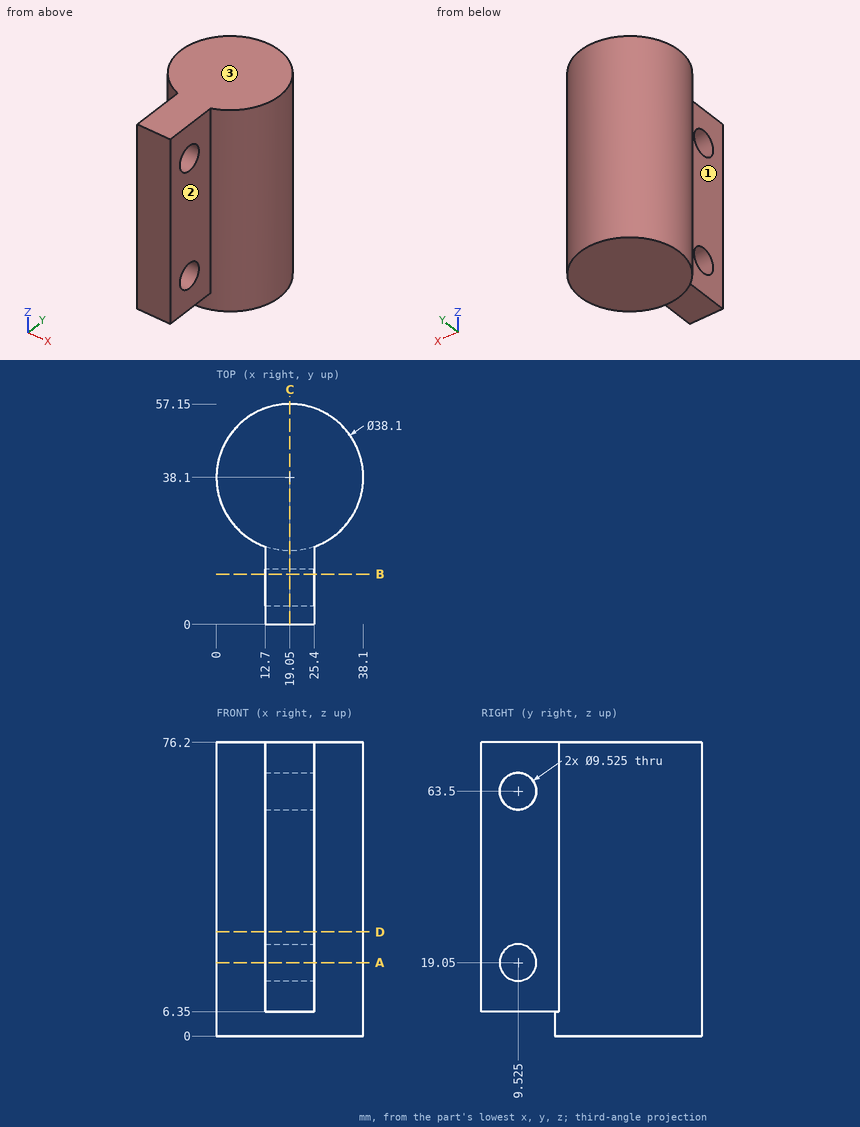
Part print with two shaded views. Sizes in mm from the minimum x, y, z corner. A direction names the side the tool comes from. Coordinates: 2 decimals unless noted, no trailing zeros. Loops run counter-clockwise (first coordinate to the right, second up) from the corner with the lowest first, then second, coordinate; pieces in that order, holes last. Notation, with made-up numbers: (39.25, 65.25) - (64.25, 65.25) arc R20 ccw to (64.25, 78.25) - close; hole circle Ø1 at (79.5, 49). An arc over 180 degrees is marked (long way). Write each question's results on one line, items separated by ' | '. Start each with the question number.
Q1. Slice it at B-B on y = 13. Give the cut face in (x, z).
Q2. Probe line 1 along Z through (x, y) = (23.5, 11); line 2 along Z through (x, y) = (13.5, 18); line 3 along Y through (x, z) = (22.25, 63.5). List the from-to ranges inside material, lowest first.
Q3. Which spindle directions (+Z, -Z, +X, -X, +Y, -Y) get a long thin tool onto all of the face, cutting with end or side? Do the marked faces 1, 2 and 3. Say none if no direction does.
Q4. Drop flat-ended pins along their axis: pin 1 Ø3 at (x, z) = (7.5, 26) entering from +Y; pin 2 Ø4 at (y, z) = (47, 8) entering from +X; pin 3 Ø12.5 at (y, z) = (9.525, 63.5) entering from -X. Give the stop position or say it passes through.
Q5. Slice it at D-D on z = 27. Give the cut face in (x, y), and give its area (3 significant figures).
Q6. Slice it at C-C on x = 19.05. Give the number of separate pieces and of enclosed holes in the cut face, and give its area (3 significant figures).
Q7. Slice it at A-A on z = 19.05. Give the cut face in (x, y), and give its area (3 significant figures).
Answer:
1) outline: (12.7, 6.35) - (25.4, 6.35) - (25.4, 15.79) - (12.7, 15.79) - close; (12.7, 22.31) - (25.4, 22.31) - (25.4, 60.24) - (12.7, 60.24) - close; (12.7, 66.76) - (25.4, 66.76) - (25.4, 76.2) - (12.7, 76.2) - close
2) line 1: z = 6.35 to 14.52, 23.58 to 58.97, 68.03 to 76.2 | line 2: z = 6.35 to 76.2 | line 3: y = 0 to 4.76, 14.29 to 56.88
3) face 1: +Z, -Z, -X, -Y | face 2: +Z, -Z, +X, -Y | face 3: +Z, +X, -X, +Y, -Y
4) pin 1: stops at y = 54.28 | pin 2: stops at x = 36.81 | pin 3: stops at x = 12.7
5) outline: (12.7, 0) - (25.4, 0) - (25.4, 20.14) arc R19.05 ccw (long way) to (12.7, 20.14) - close | area: 1,390 mm2
6) separate pieces: 1 | enclosed holes: 2 | area: 4,090 mm2
7) outline: (12.7, 0) - (25.4, 0) - (25.4, 4.76) - (12.7, 4.76) - close; (12.7, 14.29) - (25.4, 14.29) - (25.4, 20.14) arc R19.05 ccw (long way) to (12.7, 20.14) - close | area: 1,270 mm2
